Answer from the drawing. Dimensions are ordinates in mm from the lowest x, y and z of the part. Round coordinates to 2 decimals unless told otherwise and drop trailing zeros. Write each loop counter-clockwise with the first axis right and the second up, starting at its lowest first coordinate (ties: lowest second). Pieces come first, ordered by that corner, then holes.
1. Find section C-C (x = 0.4). Write down the section's boundary in (y, z).
2. Find section B-B (z = 11). Write down the section's boundary in (x, y).
3. Straight lines are drawn through the part: probe 1 along Y at (x, z) = (1.45, 11); probe 2 along Y at (x, z) = (0.35, 8.5); probe 3 along Z at (x, y) = (0.75, 15). For each, find the intervals that lie inside material, in ascending order.
4. A flat-ended cylindrical pin translates along its axis: pin 1 Ø8 at (y, z) = (12.5, 11) entering from -X. Find the tip coordinate at first contact, or state that the pin passes through.
5. Find section A-A (y = 12.5). Write down the section's boundary in (x, z).
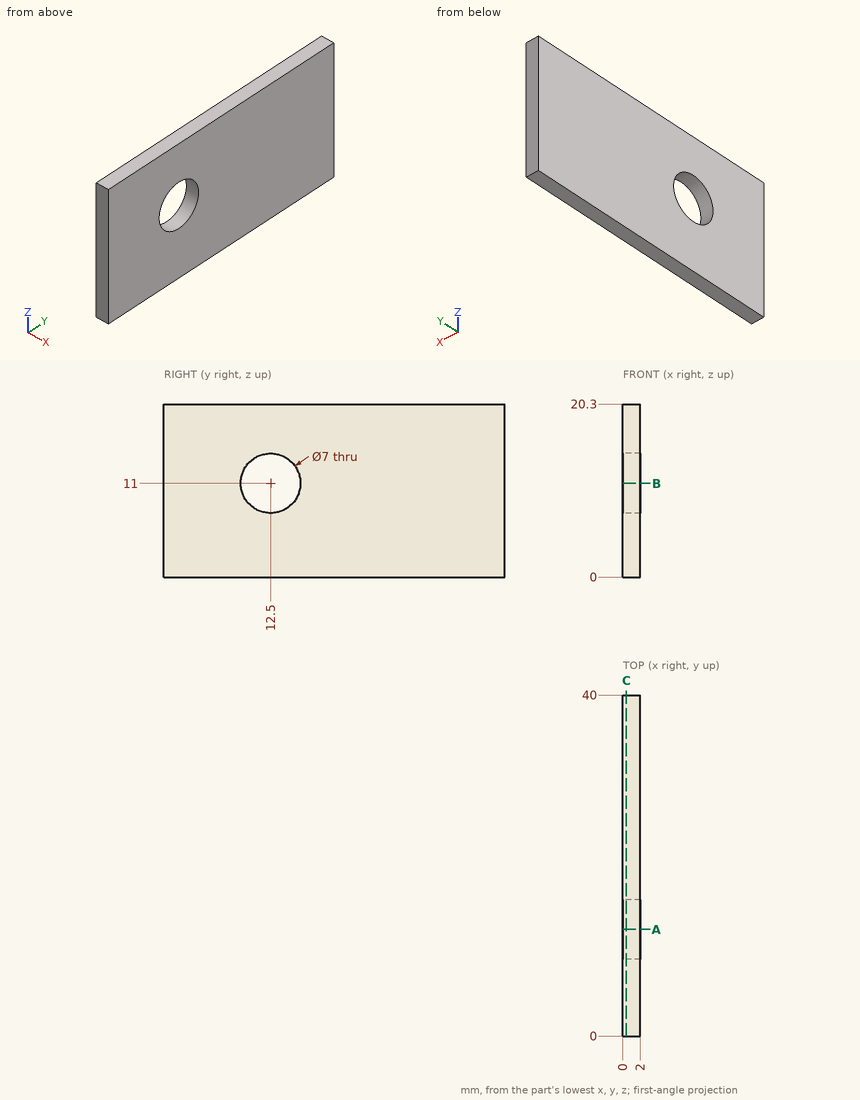
Worked answers:
1. outline: (0, 0) - (40, 0) - (40, 20.3) - (0, 20.3) - close; hole circle Ø7 at (12.5, 11)
2. outline: (0, 0) - (2, 0) - (2, 9) - (0, 9) - close; (0, 16) - (2, 16) - (2, 40) - (0, 40) - close
3. probe 1: y = 0 to 9, 16 to 40
3. probe 2: y = 0 to 10.05, 14.95 to 40
3. probe 3: z = 0 to 8.55, 13.45 to 20.3
4. pin 1: stops at x = 0
5. outline: (0, 0) - (2, 0) - (2, 7.5) - (0, 7.5) - close; (0, 14.5) - (2, 14.5) - (2, 20.3) - (0, 20.3) - close
